from build123d import *

# Parameters (mm, degrees)
F0_W     = 33.835038
F0_H     = 33.835038
F0_R     = 3.81
F1_DEPTH = 1.27
F2_R     = 1.081703
F2_R_2   = 1.08171
F3_DEPTH = 0.508


with BuildPart() as f1:
    # F0 (on Top) → F1 (new body)
    with BuildSketch(Plane.XY):
        with Locations((16.917519, 16.917519)):
            Rectangle(F0_W, F0_H)
        with Locations((16.917519, 16.917519)):
            Circle(F0_R, mode=Mode.SUBTRACT)
    extrude(amount=F1_DEPTH)

    # F2 (on face) → F3 (join)
    with BuildSketch(Plane.XY.offset(1.27)):
        with Locations((29.517038, 16.917519)):
            Circle(F2_R)
        with Locations((4.318, 16.917519)):
            Circle(F2_R)
        with Locations((16.917519, 29.517038)):
            Circle(F2_R_2)
        with Locations((16.917519, 4.318)):
            Circle(F2_R_2)
    extrude(amount=F3_DEPTH)


solid = f1.part
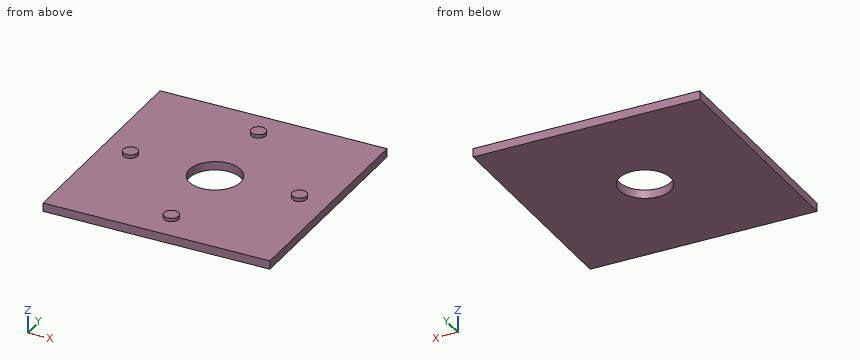
Input: part model. Units: mm. Frame: model coordinates. Coordinates: 2 decimals unless noted, no trailing zeros. Order: outer loops, then holes, each group sorted by start corner. A loop starts at its lowest first (then second) coordinate and runs counter-clockwise, first axis right, second up. Notation, with made-up numbers: M 73.25,70 L 94.25,70 A34 cw 94.25,100 Z; hole C 84.5,51 d11. An arc over 180 degrees is marked long. Write item = value, one per line. Start each with the question number.
(1) Section C-C on x = 4.5. Output: boundary loops of the cut face in (y, z).
(2) Line query: line 1 along Z through (x, y) = (9, 20); line 2 along Y through (x, z) = (14.5, 0.9); line 3 along Y through (x, z) = (15, 1). Output: solid intervals per line, ascending. Write a range as [from, to].
(3) Section B-B on x = 16.5. Output: boundary loops of the cut face in (y, z), and give its area (3 significant figures).
(4) Section D-D on y = 14. Output: boundary loops of the cut face in (x, z), and give its area (3 significant figures).
(5) Section A-A on y = 19. Output: boundary loops of the cut face in (x, z).
(6) First-contact query: P1, Ø7, axis at x = 16.92, y = 16.92, coming from the +Z side. Flat tip, straight axial feed; report the tip coordinate or a pass-through.
Result set:
q1.outline = M 0,0 L 33.84,0 L 33.84,1.27 L 17.98,1.27 L 17.98,1.78 L 15.85,1.78 L 15.85,1.27 L 0,1.27 Z
q2.line_1 = [0, 1.27]
q2.line_2 = [0, 13.97], [19.86, 33.84]
q2.line_3 = [0, 13.63], [20.21, 33.84]
q3.outline = M 0,0 L 13.13,0 L 13.13,1.27 L 5.32,1.27 L 5.32,1.78 L 3.32,1.78 L 3.32,1.27 L 0,1.27 Z; M 20.7,0 L 33.84,0 L 33.84,1.27 L 30.51,1.27 L 30.51,1.78 L 28.52,1.78 L 28.52,1.27 L 20.7,1.27 Z
q3.area = 35.4 mm²
q4.outline = M 0,0 L 14.47,0 L 14.47,1.27 L 0,1.27 Z; M 19.37,0 L 33.84,0 L 33.84,1.27 L 19.37,1.27 Z
q4.area = 36.7 mm²
q5.outline = M 0,0 L 13.73,0 L 13.73,1.27 L 0,1.27 Z; M 20.11,0 L 33.84,0 L 33.84,1.27 L 20.11,1.27 Z
q6.P1 = through
